The listing builds one solid part. Answer for the finished solid, in the listing's coordinates (mm). Give positions to 0.01 mm unless a question says otherwise; leave off trailing zeros. Loops run counter-clockwise (first coordinate to the right, second up) from the corner with the lowest first, then second, coordinate; pieces in that order, holes last. Notation, with made-up numbers: (61.25, 9) - (94.25, 9) arc R28 cw to (94.25, 33) - close; hole circle Ø9 at (57.25, 84). An arc over 180 degrees is marked (long way). Answer in a Markdown table with one row per item. Add a question column.
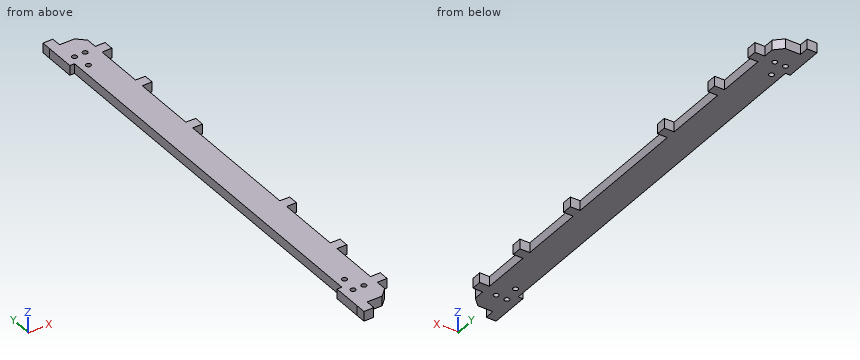
```python
from build123d import *

# Parameters (mm, degrees)
SKETCH_1_R      = 2.55
EXTRUDE_1_DEPTH = 10


with BuildPart() as part:
    # Эскиз1 → Бобышка-Вытянуть1 (new body)
    with BuildSketch(Plane.XY):
        Polygon((-16.978606932, 199), (-16.978606932, -199), (-21.7993057, -199), (-21.7993057, -229), (-21.765949224, -238.9986114), (-11.765949224, -238.9986114), (-11.5993057, -229), (3.800694299, -229), (11.800694299, -221), (11.800694299, -210.1), (21.7993057, -209.933356475), (21.7993057, -199.933356475), (11.8006943, -199.899999999), (11.8006943, -173.449999999), (11.8006943, -150.1), (21.799305701, -150.066643523), (21.799305701, -140.066643523), (11.8006943, -139.899999999), (11.8006943, -105.949999999), (11.8006943, -75.099999999), (21.7993057, -75.066643523), (21.7993057, -65.066643523), (11.8006943, -64.899999999), (11.8006943, 64.900000001), (21.7993057, 64.933356477), (21.7993057, 74.933356477), (11.8006943, 75.100000001), (11.8006943, 109.050000001), (11.8006943, 139.900000001), (21.7993057, 139.933356477), (21.7993057, 149.933356477), (11.8006943, 150.100000001), (11.8006943, 176.550000001), (11.8006943, 199.900000001), (21.7993057, 199.933356477), (21.7993057, 209.933356477), (11.8006943, 210.100000001), (11.8006943, 221), (3.8006943, 229), (-11.599305699, 229), (-11.765949224, 238.9986114), (-21.765949224, 238.9986114), (-21.7993057, 229), (-21.7993057, 199), align=None)
        with Locations((-11.199305701, -207.5)):
            Circle(SKETCH_1_R, mode=Mode.SUBTRACT)
        with Locations((-11.199305701, 207.5)):
            Circle(SKETCH_1_R, mode=Mode.SUBTRACT)
        with Locations((-0.199305701, 207.5)):
            Circle(SKETCH_1_R, mode=Mode.SUBTRACT)
        with Locations((-8.488839347, 190.647208967)):
            Circle(SKETCH_1_R, mode=Mode.SUBTRACT)
        with Locations((-0.199305701, -207.5)):
            Circle(SKETCH_1_R, mode=Mode.SUBTRACT)
        with Locations((-8.488839347, -190.65)):
            Circle(SKETCH_1_R, mode=Mode.SUBTRACT)
    extrude(amount=EXTRUDE_1_DEPTH)


solid = part.part
```
(1) Find the intervals of material crossed by line 1 along X through (y, z) = (207.5, 5); line 2 along Y through (x, z) = (-8.5, 8); line 3 along Y through (x, z) = (13, 9.25), in increasing order. Write a range as [from, to].
(2) A cutting plane is placed at B-B on z = 3.5. Give the number of separate pieces and of enclosed holes in the cut face, plus the area to 3 significant figures.
(3) A cutting plane is placed at A-A on y = -83. Determine the outline of the cut face in (x, z).
(4) Given pin 1 Ø3 at (y, z) = (-97, 4.5) entering from +X; pin 2 Ø3 at (x, y) = (-8.49, 190.65) entering from -Z; pin 3 Ø3 at (y, z) = (21.5, 7.5) entering from -X; pin 4 Ø4 at (x, z) = (-9.5, 8) entering from +Y, each flat-ended and moving along its own axis, determine where each tip first touches the part or whether it passes through.
Evaluation:
| question | item | result |
|---|---|---|
| 1 | line 1 | x = [-21.8, -13.75], [-8.65, -2.75], [2.35, 21.8] |
| 1 | line 2 | y = [-229, -193.2], [-188.1, 188.1], [193.2, 229] |
| 1 | line 3 | y = [-210.08, -199.9], [-150.1, -139.92], [-75.1, -64.92], [64.9, 75.08], [139.9, 150.08], [199.9, 210.08] |
| 2 | separate pieces | 1 |
| 2 | enclosed holes | 6 |
| 2 | area | 14,100 mm² |
| 3 | outline | (-16.98, 0) - (11.8, 0) - (11.8, 10) - (-16.98, 10) - close |
| 4 | pin 1 | stops at x = 11.8 |
| 4 | pin 2 | passes through |
| 4 | pin 3 | stops at x = -16.98 |
| 4 | pin 4 | stops at y = 229 |
